CAD build for the part. Positions are in the model's coordinates, mm. Coordinates: 2 decimals unless noted, no trailing zeros. Loops run counter-clockwise (first coordinate to the right, second up) from the corner with the lowest first, then second, coordinate; pieces in that order, holes last.
1) Saw through at A-A, the plane y = -16. Write the cut outline in (x, z).
2) Pin check, flat tip, straight feed: pin 1 Ø4 at (x, y) = (-12, -5.5) entering from -Z. Stop position of the tip, or through.
3) Saw through at B-B, the plane x = -15.5. Write the cut outline in (y, z).
4) Two-plate mould, pull along X, no slides. Class faces 1 (the flat face through (0, -18, 1)), 2 (the flat face through (-17.5, 0, 1)), 3 (the cylindrical face through (14, 16, 1)): +X half, -X half, draft (parallel to the pull), parting line (faces both ways), or undercut.
5) Wall check: line 1 along Y through (x, z) = (15.5, 1.25); line 2 along X through (y, z) = (15, 1.4). Give the ranges that are in metal, low to high.
6) Saw through at C-C, the plane z = 1.1. Write the cut outline in (x, y).
```python
from build123d import *

# Parameters (mm, degrees)
SKETCH_1_W          = 35
SKETCH_1_H          = 36
EXTRUDE_1_DEPTH     = 2
CUT_EXTRUDE_1_REACH = 27.184
SKETCH_2_R          = 1.5


with BuildPart() as part:
    # 草图1 → 凸台-拉伸1 (new body)
    with BuildSketch(Plane.XY):
        Rectangle(SKETCH_1_W, SKETCH_1_H)
    extrude(amount=EXTRUDE_1_DEPTH)

    # 草图2 → 切除-拉伸1 (cut, up to next)
    with BuildSketch(Plane.XY.offset(2), mode=Mode.PRIVATE) as cut_extrude_1_sk1:
        with Locations((-15.5, 16)):
            Circle(SKETCH_2_R)
    cut_extrude_1_tool1 = extrude(cut_extrude_1_sk1.sketch, amount=-CUT_EXTRUDE_1_REACH, mode=Mode.PRIVATE) & part.part
    # 草图2 → 切除-拉伸1 (cut, up to next)
    with BuildSketch(Plane.XY.offset(2), mode=Mode.PRIVATE) as cut_extrude_1_sk2:
        with Locations((15.5, 16)):
            Circle(SKETCH_2_R)
    cut_extrude_1_tool2 = extrude(cut_extrude_1_sk2.sketch, amount=-CUT_EXTRUDE_1_REACH, mode=Mode.PRIVATE) & part.part
    # 草图2 → 切除-拉伸1 (cut, up to next)
    with BuildSketch(Plane.XY.offset(2), mode=Mode.PRIVATE) as cut_extrude_1_sk3:
        with Locations((15.5, -16)):
            Circle(SKETCH_2_R)
    cut_extrude_1_tool3 = extrude(cut_extrude_1_sk3.sketch, amount=-CUT_EXTRUDE_1_REACH, mode=Mode.PRIVATE) & part.part
    # 草图2 → 切除-拉伸1 (cut, up to next)
    with BuildSketch(Plane.XY.offset(2), mode=Mode.PRIVATE) as cut_extrude_1_sk4:
        with Locations((-15.5, -16)):
            Circle(SKETCH_2_R)
    cut_extrude_1_tool4 = extrude(cut_extrude_1_sk4.sketch, amount=-CUT_EXTRUDE_1_REACH, mode=Mode.PRIVATE) & part.part
    add(cut_extrude_1_tool1.solids().sort_by_distance((-15.5, 16, 2))[0], mode=Mode.SUBTRACT)
    add(cut_extrude_1_tool2.solids().sort_by_distance((15.5, 16, 2))[0], mode=Mode.SUBTRACT)
    add(cut_extrude_1_tool3.solids().sort_by_distance((15.5, -16, 2))[0], mode=Mode.SUBTRACT)
    add(cut_extrude_1_tool4.solids().sort_by_distance((-15.5, -16, 2))[0], mode=Mode.SUBTRACT)


solid = part.part
```
Data:
1. outline: (-17.5, 0) - (-17, 0) - (-17, 2) - (-17.5, 2) - close; (-14, 0) - (14, 0) - (14, 2) - (-14, 2) - close; (17, 0) - (17.5, 0) - (17.5, 2) - (17, 2) - close
2. pin 1: stops at z = 0
3. outline: (-18, 0) - (-17.5, 0) - (-17.5, 2) - (-18, 2) - close; (-14.5, 0) - (14.5, 0) - (14.5, 2) - (-14.5, 2) - close; (17.5, 0) - (18, 0) - (18, 2) - (17.5, 2) - close
4. face 1: draft
4. face 2: -X half
4. face 3: undercut
5. line 1: y = -18 to -17.5, -14.5 to 14.5, 17.5 to 18
5. line 2: x = -17.5 to -16.62, -14.38 to 14.38, 16.62 to 17.5
6. outline: (-17.5, -18) - (17.5, -18) - (17.5, 18) - (-17.5, 18) - close; hole circle Ø3 at (-15.5, -16); hole circle Ø3 at (-15.5, 16); hole circle Ø3 at (15.5, -16); hole circle Ø3 at (15.5, 16)
